from build123d import *

# Parameters (mm, degrees)
SKETCH_1_W          = 50
SKETCH_1_H          = 20
EXTRUDE_1_DEPTH     = 3
SKETCH_2_W          = 50
SKETCH_2_H          = 15
EXTRUDE_2_DEPTH     = 6
SKETCH_5_W          = 50
SKETCH_5_H          = 12
CUT_EXTRUDE_2_DEPTH = 3
SKETCH_4_R          = 1.65
SKETCH_4_R_2        = 0.5
SKETCH_4_R_3        = 0.75
CUT_EXTRUDE_1_DEPTH = 3


with BuildPart() as part:
    # 草图1 → 凸台-拉伸1 (new body)
    with BuildSketch(Plane.XY):
        Rectangle(SKETCH_1_W, SKETCH_1_H)
        with BuildLine():
            Line((-5.208438024, 2.5), (5.208438024, 2.5))
            ThreePointArc((5.208438024, 2.5), (5.761208823, 2.666666667), (6.129722688, 3.111111111))
            ThreePointArc((6.129722688, 3.111111111), (21.5, 0), (6.129722688, -3.111111111))
            ThreePointArc((6.129722688, -3.111111111), (5.761208823, -2.666666667), (5.208438024, -2.5))
            Line((5.208438024, -2.5), (-5.208438024, -2.5))
            ThreePointArc((-5.208438024, -2.5), (-5.761208823, -2.666666667), (-6.129722688, -3.111111111))
            ThreePointArc((-6.129722688, -3.111111111), (-21.5, 0), (-6.129722688, 3.111111111))
            ThreePointArc((-6.129722688, 3.111111111), (-5.761208823, 2.666666667), (-5.208438024, 2.5))
        make_face(mode=Mode.SUBTRACT)
        with BuildLine():
            Line((3.25, 5.5), (-3.25, 5.5))
            ThreePointArc((-3.25, 5.5), (-5, 7.25), (-3.25, 9))
            Line((-3.25, 9), (3.25, 9))
            ThreePointArc((3.25, 9), (5, 7.25), (3.25, 5.5))
        make_face(mode=Mode.SUBTRACT)
    extrude(amount=EXTRUDE_1_DEPTH)

    # 草图2 → 凸台-拉伸2 (add)
    with BuildSketch(Plane(origin=(0, 10, 0), x_dir=(1, 0, 0), z_dir=(0, 1, 0))):
        with Locations((0, -7.5)):
            Rectangle(SKETCH_2_W, SKETCH_2_H)
    extrude(amount=EXTRUDE_2_DEPTH)

    # 草图5 → 切除-拉伸2 (cut)
    with BuildSketch(Plane.XZ.offset(-10)):
        with Locations((0, 9)):
            Rectangle(SKETCH_5_W, SKETCH_5_H)
    extrude(amount=-CUT_EXTRUDE_2_DEPTH, mode=Mode.SUBTRACT)

    # 草图4 → 切除-拉伸1 (cut)
    with BuildSketch(Plane(origin=(0, 16, 0), x_dir=(1, 0, 0), z_dir=(0, 1, 0))):
        with Locations((0, -9)):
            Circle(SKETCH_4_R)
        with Locations((6.5, -9)):
            Circle(SKETCH_4_R_2)
        with Locations((-6.5, -9)):
            Circle(SKETCH_4_R_2)
        with Locations((11, -9)):
            Circle(SKETCH_4_R_3)
        with Locations((-10.5, -9)):
            Circle(SKETCH_4_R_3)
        with Locations((0, -4.5)):
            Circle(SKETCH_4_R_2)
        with Locations((0, -13.5)):
            Circle(SKETCH_4_R_2)
    extrude(amount=-CUT_EXTRUDE_1_DEPTH, mode=Mode.SUBTRACT)


solid = part.part
Here's how the part is built. I have some questions about the finished solid (model axes, mm). A direction names the side the tool comes from. Give positions to 0.01 mm unless a question says otherwise; leave off trailing zeros. Write each loop counter-clockwise with the first axis right and the second up, starting at its lowest first coordinate (ties: lowest second). Pieces come first, ordered by that corner, then holes. Notation, with made-up numbers: (50, 42) -> (76, 42) arc R15 cw to (76, 60) -> close; hole circle Ø2 at (36, 89.25). An arc over 180 degrees is marked (long way). Use one line per item in the form item = value. Start each with the question number.
1. Will these pins go through, and if not, where does the flat tip stop? pin 1 Ø13 at (x, y) = (13.5, 0) entering from +Z; pin 2 Ø6 at (x, z) = (-10, 10) entering from -Y; pin 3 Ø2 at (x, y) = (6.5, -4.5) entering from +Z.
2. Imagine slicing it at B-B on x = 0. List the corners of the cut face in (y, z) for me, plus the area to 3 significant figures.
3. On a 3-axis mill with a long thin cutter (end or side, diameter ignored), from which of +Z, -Z, +X, -X, +Y, -Y can I reach the whole of each face in a straight line? I mean faces 4 (the face through (0, 13, 6)), 5 (the face through (0, -2.5, 1)), 6 (the face through (0, 16, 6)). Say none if no direction works.
4. Imagine slicing it at D-D on z = 9. List the corners of the cut face in (x, y) for me.
5. Imagine slicing it at A-A on y = 0. List the corners of the cut face in (x, z) for me.
6. If I drill on L1, parallel to X at y = 15.1, z = 9; L2, parallel to Z at x = 0, y = 14.1; L3, parallel to Y at x = -13.5, z = 1.05, over which ranges is the centre line in solid material (lowest first)?
7. Thinking about a two-plate mould opening in X: for faces 1 (the face through (21.494, 0.307, 1.479)), 2 (the face through (0, 14, 15)), 3 (the face through (-25, 5.8, 2.5)), which applies, +X half, -X half, draft (parallel to the pull), parting line (faces both ways), or undercut?
8. Imagine slicing it at C-C on x = 13.5. List the corners of the cut face in (y, z) for me.
Entries:
q1.pin_1 = through
q1.pin_2 = 13
q1.pin_3 = 3
q2.outline = (-10, 0) -> (-2.5, 0) -> (-2.5, 3) -> (-10, 3) -> close; (2.5, 0) -> (5.5, 0) -> (5.5, 3) -> (2.5, 3) -> close; (9, 0) -> (16, 0) -> (16, 4) -> (13, 4) -> (13, 3) -> (9, 3) -> close; (13, 5) -> (16, 5) -> (16, 7.35) -> (13, 7.35) -> close; (13, 10.65) -> (16, 10.65) -> (16, 13) -> (13, 13) -> close; (13, 14) -> (16, 14) -> (16, 15) -> (13, 15) -> close
q2.area = 72.6 mm²
q3.face_4 = +Z, +X, -X, -Y
q3.face_5 = +Z, -Z
q3.face_6 = +Z, -Z, +X, -X, +Y
q4.outline = (-25, 13) -> (-11.25, 13) -> (-11.25, 16) -> (-25, 16) -> close; (-9.75, 13) -> (-7, 13) -> (-7, 16) -> (-9.75, 16) -> close; (-6, 13) -> (-1.65, 13) -> (-1.65, 16) -> (-6, 16) -> close; (1.65, 13) -> (6, 13) -> (6, 16) -> (1.65, 16) -> close; (7, 13) -> (10.25, 13) -> (10.25, 16) -> (7, 16) -> close; (11.75, 13) -> (25, 13) -> (25, 16) -> (11.75, 16) -> close
q5.outline = (-25, 0) -> (-21.5, 0) -> (-21.5, 3) -> (-25, 3) -> close; (21.5, 0) -> (25, 0) -> (25, 3) -> (21.5, 3) -> close
q6.L1 = -25 to -11.25, -9.75 to -7, -6 to -1.65, 1.65 to 6, 7 to 10.25, 11.75 to 25
q6.L2 = 0 to 4, 5 to 7.35, 10.65 to 13, 14 to 15
q6.L3 = -10 to -8, 8 to 16
q7.face_1 = undercut
q7.face_2 = draft
q7.face_3 = -X half
q8.outline = (-10, 0) -> (-8, 0) -> (-8, 3) -> (-10, 3) -> close; (8, 0) -> (16, 0) -> (16, 15) -> (13, 15) -> (13, 3) -> (8, 3) -> close
